CAD build for the part. Positions are in the model's coordinates, mm. A direction names the side the tool comes from. Give positions to 0.01 mm unless a question says otherwise; leave off trailing zeros. Loops run counter-clockwise (first coordinate to the right, second up) from the corner with the lowest first, then second, coordinate; pieces in that order, holes last.
Item 1: Probe probe 1 along X at (y, z) = (0, -6.7); probe 2 along Y at (x, z) = (0.5, -8); probe 3 along Z at (x, y) = (5, 7.5). List the from-to ranges inside material, lowest first.
Item 2: Saw through at A-A on y = 3.25. Give the cut face in (x, z), plus the area to 3 significant figures.
Item 3: Mould opens along Y. For faces 1 (the cylindrical face through (4.93, 7.71, -1.95)), 2 (the flat face through (6.5, 0.9, -1)), 3 (the flat face through (6.8, 1, -1)) say: released by +Y, released by -Y, zero draft, split by the parting line, or undercut.
Item 4: Saw through at C-C on y = -2. Give the cut face in (x, z), plus the area to 3 significant figures.
Item 5: Saw through at B-B on z = -3.5. Give the cut face in (x, y).
Item 6: Which spindle directions (+Z, -Z, +X, -X, +Y, -Y) get a long thin tool onto all of the face, cutting with end or side? Do faces 4 (the cylindrical face through (4.93, -3.42, -7.18)), 5 (the cylindrical face through (0.84, 1.07, -1.05)), 6 (the flat face through (5, -4, -1.5)). Say none if no direction does.
Item 7: Drop flat-ended pins along their axis: P1, Ø4, axis at x = 8.5, y = -5.5, coming from the +Z side; P2, Ø6, axis at x = 5.5, y = -5, coming from the -Z side; P3, Ø4, axis at x = 4.5, y = 4.5, coming from the +Z side; P4, Ø1, axis at x = 6, z = -3, coming from the -Y side. Give the stop position or say it passes through.
from build123d import *

# Parameters (mm, degrees)
BASPROSKE_W             = 10
BASPROSKE_H             = 8.5
TOOTHCUT_DEPTH          = 16.636495771
TEETHCUTS_COUNT         = 32
BORSKE_R                = 1
BORE_DEPTH              = 50.0000508
SKETCH1_R               = 2.25
CUT_EXTRUDE1_DEPTH      = 3.2
SKETCH2_W               = 3
SKETCH2_H               = 10
CUT_EXTRUDE2_DEPTH      = 16.610070769
CUT_EXTRUDE3_DEPTH      = 17.472745672
CUT_EXTRUDE3_DEPTH_BACK = 17.472745672
SKETCH3_R               = 0.6
SKETCH4_R               = 1.5
CUT_EXTRUDE4_DEPTH      = 6.5
SKETCH7_W               = 10.973728646
SKETCH7_H               = 17.598113622
CUT_EXTRUDE5_DEPTH      = 10
SKETCH8_W               = 2.7
SKETCH8_H               = 3.7
CUT_EXTRUDE6_DEPTH      = 2.2


with BuildPart() as part:
    # BasProSke → Base-Revolve (revolve)
    with BuildSketch(Plane(origin=(0, 0, 0), x_dir=(1, 0, 0), z_dir=(0, 1, 0)), mode=Mode.PRIVATE) as base_revolve_sk:
        with Locations((5, 4.25)):
            Rectangle(BASPROSKE_W, BASPROSKE_H)
    revolve(base_revolve_sk.sketch.rotate(Axis((-10, 0, 0), (1, 0, 0)), 180), axis=Axis((-10, 0, 0), (1, 0, 0)))

    # TooCutSke → ToothCut (cut, through all)
    with BuildSketch(Plane(origin=(0, 0, 0), x_dir=(0, 0, -1), z_dir=(1, 0, 0))):
        with BuildLine():
            ThreePointArc((0.277002447, 7.3687954), (0, 7.374), (-0.277002447, 7.3687954))
            ThreePointArc((-0.277002447, 7.3687954), (-0.41335061, 7.952280695), (-0.656086882, 8.500117362))
            ThreePointArc((-0.656086882, 8.500117362), (0, 8.5254), (0.656086882, 8.500117362))
            ThreePointArc((0.656086882, 8.500117362), (0.41335061, 7.952280695), (0.277002447, 7.3687954))
        make_face()
    toothcut = extrude(amount=TOOTHCUT_DEPTH, mode=Mode.SUBTRACT)

    # TeethCuts: ToothCut ×32 about axis
    teethcuts_axis = Axis((0, 0, 0), (1, 0, 0))
    for i in range(1, TEETHCUTS_COUNT):
        add(toothcut.rotate(teethcuts_axis, i * 360 / TEETHCUTS_COUNT), mode=Mode.SUBTRACT)

    # BorSke → Bore (cut, symmetric)
    with BuildSketch(Plane(origin=(0, 0, 0), x_dir=(0, 0, -1), z_dir=(1, 0, 0))):
        with Locations(Location((0, 0, 0), (0, 0, 180))):
            Circle(BORSKE_R)
    extrude(amount=BORE_DEPTH, both=True, mode=Mode.SUBTRACT)

    # Sketch1 → Cut-Extrude1 (cut)
    with BuildSketch(Plane(origin=(10, 0, 0), x_dir=(0, 0, -1), z_dir=(1, 0, 0))):
        Circle(SKETCH1_R)
    extrude(amount=-CUT_EXTRUDE1_DEPTH, mode=Mode.SUBTRACT)

    # Sketch2 → Cut-Extrude2 (cut, through all)
    with BuildSketch(Plane.ZY):
        with Locations((0, -5)):
            Rectangle(SKETCH2_W, SKETCH2_H)
    extrude(amount=-CUT_EXTRUDE2_DEPTH, mode=Mode.SUBTRACT)

    # Sketch3 → Cut-Extrude3 (cut, two sides: drawn at the far end of the back side and taken through both)
    with BuildSketch(Plane.XY.offset(-1.5).offset(-CUT_EXTRUDE3_DEPTH_BACK)):
        with Locations((4, 0)):
            Circle(SKETCH3_R)
    extrude(amount=CUT_EXTRUDE3_DEPTH + CUT_EXTRUDE3_DEPTH_BACK, mode=Mode.SUBTRACT)

    # Sketch4 → Cut-Extrude4 (cut)
    with BuildSketch(Plane.ZY):
        Circle(SKETCH4_R)
    extrude(amount=-CUT_EXTRUDE4_DEPTH, mode=Mode.SUBTRACT)

    # Sketch6 → Cut-Revolve1 (revolve, cut)
    with BuildSketch(Plane.XY):
        with BuildLine():
            ThreePointArc((4, 2.75), (6.75, 0), (4, -2.75))
            Line((4, -2.75), (4, 0))
            Line((4, 0), (4, 2.75))
        make_face()
    revolve(axis=Axis((4, 0, 0), (0, -1, 0)), mode=Mode.SUBTRACT)

    # Sketch7 → Cut-Extrude5 (cut)
    with BuildSketch(Plane.XY):
        with Locations((4.910782694, 0.110648149)):
            Rectangle(SKETCH7_W, SKETCH7_H)
    extrude(amount=CUT_EXTRUDE5_DEPTH, mode=Mode.SUBTRACT)

    # Sketch8 → Cut-Extrude6 (cut)
    with BuildSketch(Plane.XY):
        with Locations((7.35, 4.7)):
            Rectangle(SKETCH8_W, SKETCH8_H)
        with Locations((2.85, 4.7)):
            Rectangle(SKETCH8_W, SKETCH8_H)
    extrude(amount=-CUT_EXTRUDE6_DEPTH, mode=Mode.SUBTRACT)


solid = part.part
Results below:
1. probe 1: x = 0 to 3.4, 4.6 to 10
1. probe 2: y = -2.66 to -2.14, -1.13 to -0.43, 0.43 to 1.13, 2.14 to 2.66
1. probe 3: z = -4 to -3.74, -2.66 to -1.84, -1.17 to -0.3
2. outline: (0, -6.97) - (10, -6.97) - (10, 0) - (8.7, 0) - (8.7, -2.2) - (6, -2.2) - (6, 0) - (4.2, 0) - (4.2, -2.2) - (1.5, -2.2) - (1.5, 0) - (0, 0) - close
2. area: 57.8 mm2
3. face 1: released by +Y
3. face 2: zero draft
3. face 3: undercut
4. outline: (0, -7.79) - (10, -7.79) - (10, -1.5) - (5.15, -1.5) arc R1.89 cw to (2.85, -1.5) - (0, -1.5) - close
4. area: 62.3 mm2
5. outline: (0, -7.27) - (10, -7.27) - (10, 7.27) - (0, 7.27) - close; hole circle Ø1.2 at (4, 0)
6. face 4: -Z, +X, -X
6. face 5: +Z, -X, -Y
6. face 6: +Z, +X, -X, -Y
7. P1: stops at z = -1.5
7. P2: stops at z = -8.19
7. P3: stops at z = 0
7. P4: stops at y = -8.12
